Work out the finished part from the listing and answer in its coordinate system (mm). A direction names the side the tool comes from. Coordinates: 2 decimals unless noted, no trailing zeros. Write each loop counter-clockwise with the first axis right and the second up, starting at its lowest first coordinate (ties: lowest second). Pieces come first, ordered by that corner, then holes. Notation, with made-up numbers: (5, -30) - (56, -30) arc R25 ccw to (56, 9) - close; hole circle Ø5 at (7.5, 42). An arc over 180 degrees is marked (long way). Use a Markdown table: item, result. Add a question column.
(1) Find the intervals of material crossed by line 1 (Z direction, x = -1, y = 110); line 2 (Z direction, x = 4, y = 110); line 3 (Y direction, x = 18, z = -4.5), in increasing order. Write a range as from..to.
(2) A tool of negligible diameter and unlimited length cuts with its end or side. For faces 1 (the face through (10.68, 104.24, 3.52)), 2 (the face through (10, -15, 0)), 3 (the face through (14.872, 74, 0)), 4 (the face through (-5.478, 135, 0)), 5 (the face through (0.522, 111.93, 4.23)), from which of +Z, -Z, +X, -X, +Y, -Y can it reach the whole face along a straight path? Write none if from no direction.
(3) The part is cut by section B-B, the plane y = 97. Give the vertices of the cut face in (x, z).
(4) The part is cut by section A-A, the plane x = 4.5. Give the vertices of the cut face in (y, z).
(5) The part is cut by section C-C, the plane x = 20. Give the vertices of the cut face in (y, z).
(6) Given pin 1 Ø4 at (y, z) = (107, 1.5) entering from +X; pin 2 Ø5 at (y, z) = (4, -3.5) entering from -X, each flat-ended and moving along its own axis, determine where each tip first touches the part or whether it passes through.
Autodesk Inventor part; units mm, degrees
ref_plane "YZ Plane" through (0, 0, 0) normal (1, 0, 0) x (0, 1, 0)
ref_plane "XZ Plane" through (0, 0, 0) normal (0, 1, 0) x (-1, 0, 0)
ref_plane "XY Plane" through (0, 0, 0) normal (0, 0, 1) x (1, 0, 0)
sketch "Sketch1" plane through (0, 0, 0) normal (0, 1, 0) x (-1, 0, 0)
  line L0 (5.4777, 10.4253) -> (-14.8723, 10.4253)
  line L1 (-14.8723, 10.4253) -> (-14.8723, -9.9247)
  line L2 (-14.8723, -9.9247) -> (5.4777, -9.9247)
  line L3 (5.4777, -9.9247) -> (5.4777, 10.4253)
  point P0 (0, 0)
  dimension "d0" = 20.35
  dimension "d1" = 20.35
extrude "Extrusion1" add sketch "Sketch1" along normal blind 150
fillet "Fillet1" radius 1 4 edges at (14.8723, 75, 10.4253) (14.8723, 75, -9.9247) (-5.4777, 75, 10.4253) (-5.4777, 75, -9.9247)
sketch "Sketch2" plane through (14.8723, 0, 9.4253) normal (1, 0, 0) x (0, 0, -1)
  line L0 (9.175, 102.3501) -> (2.55, 106.1751)
  line L1 (2.55, 106.1751) -> (2.55, 113.8249)
  line L2 (2.55, 113.8249) -> (9.175, 117.6499)
  line L3 (9.175, 117.6499) -> (15.8, 113.8249)
  line L4 (15.8, 113.8249) -> (15.8, 106.1751)
  line L5 (15.8, 106.1751) -> (9.175, 102.3501)
  line L6 (18.35, 150) -> (18.35, 0)
  line L7 (0, 150) -> (18.35, 150)
  line L8 (0, 0) -> (0, 150)
  line L9 (0, 0) -> (18.35, 0)
  line L10 (-1, 150) -> (-1, 0)
  point P0 (9.4253, 0)
  point P1 (9.175, 110)
  dimension "d5" = 13.25
  dimension "d6" = 0
  dimension "d37" = 110
  dimension "d39" = 40
  dimension "d40" = 10.175
extrude "Extrusion2" cut sketch "Sketch2" against normal blind 8.5 contours L0 L1 L2 L3 L4 L5
sketch "Sketch3" plane through (-5.4777, 0, -8.9247) normal (-1, 0, 0) x (0, 0, 1)
  circle A0 centre (9.175, 110) radius 9.25
  line L0 (0, 150) -> (18.35, 150)
  line L1 (19.35, 0) -> (19.35, 150)
  line L2 (0, 0) -> (18.35, 0)
  point P0 (8.9247, 0)
  dimension "d12" = 18.5
  dimension "d13" = 10.175
  dimension "d38" = 110
hole "Hole1" at (-5.4777, 110, 0.2503) direction (1, 0, 0) diameter 8.5 depth 40 counterbore diameter 18.5 counterbore depth 6
sketch "Sketch4" plane through (0, 0, 0) normal (0, -1, 0) x (1, 0, 0)
  line L0 (29.2223, -9.9247) -> (-8.8277, -9.9247)
  line L1 (-8.8277, -9.9247) -> (-8.8277, 10.4253)
  line L2 (-8.8277, 10.4253) -> (29.2223, 10.4253)
  line L3 (29.2223, 10.4253) -> (29.2223, -9.9247)
  line L4 (13.8723, -9.9247) -> (-4.4777, -9.9247)
  line L5 (14.8723, 9.4253) -> (14.8723, -8.9247)
  line L6 (-5.4777, -8.9247) -> (-5.4777, 9.4253)
  point P0 (0, 0)
  dimension "d22" = 20.35
  dimension "d23" = 0
  dimension "d25" = 3.35
  dimension "d36" = 14.35
extrude "Extrusion3" add sketch "Sketch4" along normal blind 15
properties part number "shaft4V1"
Model answer:
| question | item | result |
|---|---|---|
| 1 | line 1 | -9.92..-9, 9.5..10.43 |
| 1 | line 2 | -9.92..-4, 4.5..10.43 |
| 1 | line 3 | -15..0 |
| 2 | face 1 | +X |
| 2 | face 2 | +Z, -Z, +X, -X, -Y |
| 2 | face 3 | +Z, -Z, +X, +Y |
| 2 | face 4 | +Z, -Z, -X, +Y |
| 2 | face 5 | -X |
| 3 | outline | (-5.48, -8.92) arc R1 ccw to (-4.48, -9.92) - (13.87, -9.92) arc R1 ccw to (14.87, -8.92) - (14.87, 9.43) arc R1 ccw to (13.87, 10.43) - (-4.48, 10.43) arc R1 ccw to (-5.48, 9.43) - close |
| 4 | outline | (-15, -9.92) - (150, -9.92) - (150, 10.43) - (-15, 10.43) - close; hole circle Ø8.5 at (110, 0.25) |
| 5 | outline | (-15, -9.92) - (0, -9.92) - (0, 10.43) - (-15, 10.43) - close |
| 6 | pin 1 | x = 6.37 |
| 6 | pin 2 | x = -5.48 |
